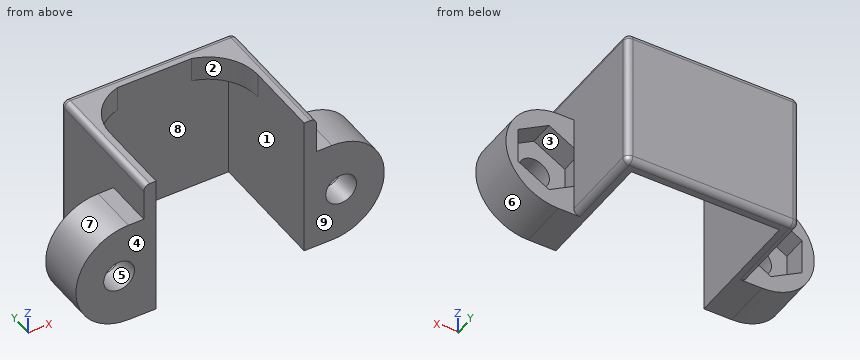
```python
from build123d import *

# Parameters (mm, degrees)
P_IDAT_VYSUNUT_M1_DEPTH  = 11.5
SKICA3_OUTSIDE_W         = 32.928
SKICA3_OUTSIDE_H         = 19.428
ODEBRAT_VYSUNUT_M1_DEPTH = 19.371173071
SKICA4_R                 = 1.25
ODEBRAT_VYSUNUT_M2_DEPTH = 19.371173071
ODEBRAT_VYSUNUT_M3_DEPTH = 2
P_IDAT_VYSUNUT_M2_DEPTH  = 2
ZAOBLIT2_R               = 0.5


with BuildPart() as part:
    # Skica1 → Přidat vysunutím1 (new body)
    with BuildSketch(Plane.XY):
        Polygon((-12.5, 0), (-6, 0), (-6, 10), (6, 10), (6, 0), (12.5, 0), (12.5, 4), (7, 4), (7, 11), (-7, 11), (-7, 4), (-12.5, 4), align=None)
    extrude(amount=P_IDAT_VYSUNUT_M1_DEPTH)

    # Skica3 outside → Odebrat vysunutím1 (cut, through all)
    with BuildSketch(Plane(origin=(0, 4, 0), x_dir=(1, 0, 0), z_dir=(0, 1, 0))):
        with Locations((0, -5.75)):
            Rectangle(SKICA3_OUTSIDE_W, SKICA3_OUTSIDE_H)
        with BuildLine():
            Line((-8.25, 0), (-7, 0))
            Line((-7, 0), (7, 0))
            Line((7, 0), (8.25, 0))
            ThreePointArc((8.25, 0), (12.5, -4.25), (8.25, -8.5))
            Line((8.25, -8.5), (7, -8.5))
            Line((7, -8.5), (7, -11.5))
            Line((7, -11.5), (-7, -11.5))
            Line((-7, -11.5), (-7, -8.5))
            Line((-7, -8.5), (-8.25, -8.5))
            ThreePointArc((-8.25, -8.5), (-12.5, -4.25), (-8.25, 0))
        make_face(mode=Mode.SUBTRACT)
    extrude(amount=-ODEBRAT_VYSUNUT_M1_DEPTH, mode=Mode.SUBTRACT)

    # Skica4 → Odebrat vysunutím2 (cut, through all)
    with BuildSketch(Plane(origin=(0, 4, 0), x_dir=(1, 0, 0), z_dir=(0, 1, 0))):
        with Locations(Location((-9, -4.25, 0), (0, 0, 270))):
            Circle(SKICA4_R)
        with Locations(Location((9, -4.25, 0), (0, 0, 90))):
            Circle(SKICA4_R)
    extrude(amount=-ODEBRAT_VYSUNUT_M2_DEPTH, mode=Mode.SUBTRACT)

    # Skica5 → Odebrat vysunutím3 (cut)
    with BuildSketch(Plane(origin=(0, 4, 0), x_dir=(1, 0, 0), z_dir=(0, 1, 0))):
        Polygon((-6.5, -5.693375673), (-6.5, -2.806624327), (-9, -1.363248654), (-11.5, -2.806624327), (-11.5, -5.693375673), (-9, -7.136751346), align=None)
        Polygon((9, -7.136751346), (6.5, -5.693375673), (6.5, -2.806624327), (9, -1.363248654), (11.5, -2.806624327), (11.5, -5.693375673), align=None)
    extrude(amount=-ODEBRAT_VYSUNUT_M3_DEPTH, mode=Mode.SUBTRACT)

    # Skica6 → Přidat vysunutím2 (add)
    with BuildSketch(Plane.XY.offset(11.5)):
        with BuildLine():
            Line((-6, 10), (-3, 10))
            ThreePointArc((-3, 10), (-5.16227766, 8.576506397), (-6, 6.127016654))
            Line((-6, 6.127016654), (-6, 10))
        make_face()
        with BuildLine():
            Line((6, 6.127016654), (6, 10))
            Line((6, 10), (3, 10))
            ThreePointArc((3, 10), (5.16227766, 8.576506397), (6, 6.127016654))
        make_face()
    extrude(amount=-P_IDAT_VYSUNUT_M2_DEPTH)

    # Zaoblit2
    zaoblit2_edges = [part.edges().sort_by_distance(p)[0] for p in [
        (-7, 7.5, 0),
        (0, 11, 0),
        (7, 7.5, 0),
        (-7, 11, 5.75),
        (7, 11, 5.75),
        (7, 5.5, 11.5),
        (0, 11, 11.5),
        (-7, 5.5, 11.5),
    ]]
    fillet(zaoblit2_edges, radius=ZAOBLIT2_R)


solid = part.part
```
The listing builds one solid part. Answer for the finished solid, in the listing's coordinates (mm). Face numbers are marked on the shaded views. A direction names the side the tool comes from. Give positions to 0.01 mm unless a question says otherwise; leave off trailing zeros. Order: outer loops, then holes, each group sorted by start corner. A loop starts at its lowest first (then second) coordinate and runs counter-clockwise, first axis right, second up.
Item 1: Which of the six approach directions +Z, -Z, +X, -X, +Y, -Y give full straight-line access (tool end or side, diameter ignored) to the marked faces 1, 2, 3, 4 and 5?
From the geometry:
face 1: -Z, -Y
face 2: +Z, -Z, -Y
face 3: none
face 4: +Z, -Z, +X, -X, -Y
face 5: +Y, -Y
Item 2: The part is cut by section A-A, the plane y = 2.75. Give the vertices of the cut face in (x, z).
From the geometry:
outline: (-8.25, 0) - (-6, 0) - (-6, 11.5) - (-6.5, 11.5) arc R0.5 ccw to (-7, 11) - (-7, 8.5) - (-8.25, 8.5) arc R4.25 ccw to start; (6, 0) - (8.25, 0) arc R4.25 ccw to (8.25, 8.5) - (7, 8.5) - (7, 11) arc R0.5 ccw to (6.5, 11.5) - (6, 11.5) - close; hole (-11.5, 2.81) - (-9, 1.36) - (-6.5, 2.81) - (-6.5, 5.69) - (-9, 7.14) - (-11.5, 5.69) - close; hole (6.5, 2.81) - (9, 1.36) - (11.5, 2.81) - (11.5, 5.69) - (9, 7.14) - (6.5, 5.69) - close
Item 3: The part is cut by section B-B, the plane y = 5.5. Give the vertices of the cut face in (x, z).
From the geometry:
outline: (-7, 0.5) arc R0.5 ccw to (-6.5, 0) - (-6, 0) - (-6, 11.5) - (-6.5, 11.5) arc R0.5 ccw to (-7, 11) - close; (6, 0) - (6.5, 0) arc R0.5 ccw to (7, 0.5) - (7, 11) arc R0.5 ccw to (6.5, 11.5) - (6, 11.5) - close
Item 4: The part is cut by section C-C, the plane z = 4.25. Count the separate pieces of the cut face and the enclosed holes in it, and give its area (3 significant figures).
From the geometry:
separate pieces: 3
enclosed holes: 0
area: 47.9 mm2
Item 5: For a pull along X with two mould halves and no side action, classify the marked faces 6, 7, 8 and 9 as pulls with the +X half, pulls with the -X half, needs draft (parallel to the pull), parting line crosses it, or undercut.
From the geometry:
face 6: pulls with the +X half
face 7: pulls with the -X half
face 8: undercut
face 9: needs draft
Item 6: Given pin 1 Ø0.6 at (x, y) = (7.5, 2.5) entering from +Z; pin 2 Ø1.5 at (x, y) = (-5, 8.5) entering from -Z; pin 3 Ø1.5 at (x, z) = (9, 4.25) entering from -Y (1 decimal); pin 4 Ø1.5 at (y, z) = (3.5, 10) entering from -X, each flat-ended and moving along its own axis, determine where each tip first touches the part or whether it passes through.
From the geometry:
pin 1: stops at z = 8.5
pin 2: stops at z = 9.5
pin 3: passes through
pin 4: stops at x = -7
Item 7: Find the intervals of material crossed by probe 1 along X at (y, z) = (1.1, 4.25); probe 2 along X at (y, z) = (8.25, 1.25); probe 3 along Y at (x, z) = (-9.75, 7), in increasing order.
From the geometry:
probe 1: x = -12.5 to -10.25, -7.75 to -6, 6 to 7.75, 10.25 to 12.5
probe 2: x = -7 to -6, 6 to 7
probe 3: y = 0 to 4
Item 8: The part is cut by section D-D, the plane x = 6.75. Give the vertices of the cut face in (y, z), and give its area (3 significant figures).
From the geometry:
outline: (0, 0) - (4, 0) - (4, 0.07) - (10.5, 0.07) arc R0.43 ccw to (10.93, 0.5) - (10.93, 11) arc R0.43 ccw to (10.5, 11.43) - (0, 11.43) - close; hole (2, 2.66) - (4, 2.66) - (4, 5.84) - (2, 5.84) - close
area: 118 mm2
